Design review of the part built by this model. Coordinates are the model's own, in mm. Face numbers are marked on the shaded views. Coordinates: 2 decimals unless noted, no trailing zeros. Loops run counter-clockwise (first coordinate to the right, second up) from the corner with the lowest first, then second, coordinate; pieces in that order, holes last. Notation, with made-up numbers: (-18.5, -8.75) -> (35.5, -8.75) arc R36 ccw to (35.5, 28.25) -> close; hole circle Ø10 at (79, -34). An arc over 180 degrees is marked (long way). Answer in a Markdown table with one row per item.
Autodesk Inventor part; units mm, degrees
ref_plane "YZ Plane" through (0, 0, 0) normal (1, 0, 0) x (0, 1, 0)
ref_plane "XZ Plane" through (0, 0, 0) normal (0, 1, 0) x (-1, 0, 0)
ref_plane "XY Plane" through (0, 0, 0) normal (0, 0, 1) x (1, 0, 0)
sketch "Sketch1" plane through (0, 0, 0) normal (0, 1, 0) x (-1, 0, 0)
  circle A0 centre (0, 0) radius 10.5
  line L0 (0, 0) -> (0, -23.5)
  circle A1 centre (0, -23.5) radius 5.25
  line L1 (0, -23.5) -> (0, -35.25)
  line L2 (-14, -35.25) -> (-14, -58.75)
  line L3 (-14, -58.75) -> (-19, -58.75)
  line L4 (-19, -58.75) -> (-19, -35.25)
  line L5 (-36.5, 21.625) -> (34, 21.625)
  line L6 (-36.5, 21.625) -> (34, 21.625) construction
  line L7 (34, 21.625) -> (24, 21.625)
  line L8 (-36.5, 21.625) -> (34, 21.625)
  line L9 (34, 21.625) -> (34, -69.875)
  line L10 (34, -69.875) -> (-36.5, -69.875)
  line L11 (-36.5, -69.875) -> (-36.5, 21.625)
  line L12 (-36.5, 21.625) -> (-36.5, 11.625)
  line L13 (-36.5, 11.625) -> (-26.5, 11.625)
  circle A2 centre (-26.5, 11.625) radius 3.5
  line L14 (34, 21.625) -> (24, 21.625)
  line L15 (24, 21.625) -> (24, 11.625)
  circle A3 centre (24, 11.625) radius 3.5
  line L16 (34, -69.875) -> (24, -69.875)
  line L17 (24, -69.875) -> (24, -59.875)
  circle A4 centre (24, -59.875) radius 3.5
  line L18 (-36.5, -69.875) -> (-26.5, -69.875)
  line L19 (-26.5, -69.875) -> (-26.5, -59.875)
  circle A5 centre (-26.5, -59.875) radius 3.5
  line L20 (-26.5, 11.625) -> (-26.5, -18.375)
  line L21 (24, -59.875) -> (24, -29.875)
  circle A6 centre (-26.5, -18.375) radius 2.5
  circle A7 centre (24, -29.875) radius 2.5
  line L22 (-19, -35.25) -> (-14, -35.25)
  dimension "d0" = 21
  dimension "d1" = 23.5
  dimension "d2" = 10.5
  dimension "d3" = 11.75
  dimension "d5" = 23.5
  dimension "d6" = 5
  dimension "d7" = 23.5
  dimension "d9" = 70.5
  dimension "d40" = 21.625
  dimension "d41" = 70.5
  dimension "d42" = 91.5
  dimension "d43" = 10
  dimension "d44" = 10
  dimension "d45" = 7
  dimension "d46" = 10
  dimension "d47" = 10
  dimension "d48" = 90
  dimension "d50" = 7
  dimension "d51" = 10
  dimension "d52" = 10
  dimension "d53" = 7
  dimension "d54" = 10
  dimension "d55" = 10
  dimension "d56" = 7
  dimension "d60" = 30
  dimension "d61" = 30
  dimension "d62" = 5
  dimension "d63" = 5
  dimension "d64" = 14
  dimension "d121" = 34
extrude "Extrusion1" add sketch "Sketch1" along normal blind 24
hole "Hole1" at (-24, 24, -59.875) direction (0, -1, 0) diameter 3 end through all counterbore diameter 10 counterbore depth 7
hole "Hole2" at (26.5, 24, -59.875) direction (0, -1, 0) diameter 3 end through all counterbore diameter 10 counterbore depth 7
hole "Hole3" at (-24, 24, 11.625) direction (0, -1, 0) diameter 3 end through all counterbore diameter 10 counterbore depth 7
hole "Hole4" at (26.5, 24, 11.625) direction (0, -1, 0) diameter 3 end through all counterbore diameter 10 counterbore depth 7
chamfer "Chamfer1" distance 0.698 distance2 20 1 edges at (10.5, 0, 0) measured on face at (-2.5112, 0, -48.5701)
chamfer "Chamfer2" distance 0.698 distance2 20 1 edges at (5.25, 0, -23.5) measured on face at (-2.5112, 0, -48.5701)
chamfer "Chamfer3" distance 0.698 distance2 20 1 edges at (16.5, 0, -35.25) measured on face at (-2.5393, 0, -48.801)
chamfer "Chamfer4" distance 20 distance2 0.698 1 edges at (14, 0, -47) measured on face at (14, 14.6667, -50.9167)
chamfer "Chamfer5" distance 0.698 distance2 20 1 edges at (19, 0, -47) measured on face at (-2.772, 0, -48.801)
chamfer "Chamfer6" distance 0.698 distance2 20 1 edges at (16.5, 0, -58.75) measured on face at (-2.772, 0, -48.801)
properties part number "Matriz"
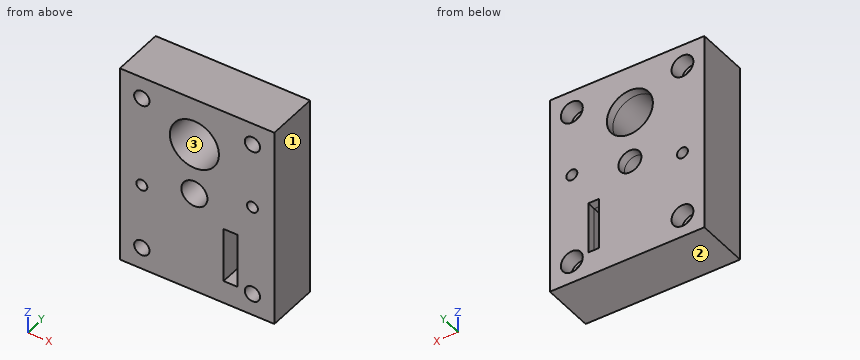
(1) For pin 1 (8 mm diameter, centred on x = -24, z = 11.625, fed in from -Y); pin 2 (3 mm diameter, centred on x = -26, z = -62, fed in from +Y), all flat-tipped, find the tip position at first contact; note any pin that passes through.
Evaluation:
| item | result |
|---|---|
| pin 1 | stops at y = 0 |
| pin 2 | stops at y = 17 |
(2) Take a section at B-B on z = -47.5. Give the boundary of the cut face in (x, y).
Evaluation:
| item | result |
|---|---|
| outline | (-34, 0) -> (13.3, 0) -> (14, 20) -> (14, 24) -> (-34, 24) -> close; (19, 20) -> (19.7, 0) -> (36.5, 0) -> (36.5, 24) -> (19, 24) -> close |
(3) Draft analysis for pull direction Z (two halves, no side actions). For the marked faces 1, 2 and 3, state which applies: pulls with the +Z half, pulls with the -Z half, needs draft (parallel to the pull), parting line crosses it, or undercut.
Evaluation:
| item | result |
|---|---|
| face 1 | needs draft |
| face 2 | pulls with the -Z half |
| face 3 | undercut |
(4) Take a section at A-A on x = 26.5. Give the boundary of the cut face in (y, z) (3 decimals).
Evaluation:
| item | result |
|---|---|
| outline | (0, -69.875) -> (24, -69.875) -> (24, -64.875) -> (17, -64.875) -> (17, -63.375) -> (0, -63.375) -> close; (0, -56.375) -> (17, -56.375) -> (17, -54.875) -> (24, -54.875) -> (24, -20.875) -> (0, -20.875) -> close; (0, -15.875) -> (24, -15.875) -> (24, 6.625) -> (17, 6.625) -> (17, 8.125) -> (0, 8.125) -> close; (0, 15.125) -> (17, 15.125) -> (17, 16.625) -> (24, 16.625) -> (24, 21.625) -> (0, 21.625) -> close |
(5) Take a section at D-D on z = -23.5. Give the boundary of the cut face in (x, y), and give its area (3 significant figures).
Evaluation:
| item | result |
|---|---|
| outline | (-34, 0) -> (-5.95, 0) -> (-5.25, 20) -> (-5.25, 24) -> (-34, 24) -> close; (5.25, 20) -> (5.95, 0) -> (36.5, 0) -> (36.5, 24) -> (5.25, 24) -> close |
| area | 1,430 mm² |
(6) Take a section at C-C on y = 4.25. Count the separate pieces of the cut face and the enclosed holes in it, and give its area (3 significant figures).
Evaluation:
| item | result |
|---|---|
| separate pieces | 1 |
| enclosed holes | 9 |
| area | 5,620 mm² |
(7) To check wall thickness, follow probe 1 along Z at (x, y) = (0, 22.95) (3 decimals); probe 2 along Z at (x, y) = (26.5, 9.75) (3 decimals); probe 3 along Z at (x, y) = (-24, 19) (3 decimals). State the ranges of each line that lie inside material, in increasing order.
Evaluation:
| item | result |
|---|---|
| probe 1 | z = -69.875 to -28.75, -18.25 to -10.5, 10.5 to 21.625 |
| probe 2 | z = -69.875 to -63.375, -56.375 to -20.875, -15.875 to 8.125, 15.125 to 21.625 |
| probe 3 | z = -69.875 to -64.875, -54.875 to -32.375, -27.375 to 6.625, 16.625 to 21.625 |
